Work out the finished part from the listing and answer in its coordinate system (mm). Give positions to 0.01 mm unless a question says otherwise; leave off trailing zeros. Loops run counter-clockwise (first coordinate to the right, second up) from the corner with the lowest first, then second, coordinate; pieces in that order, holes last. Notation, with made-up numbers: M 15.25,81.5 L 70.25,81.5 A8 cw 70.25,93.5 Z; hole C 55,15.25 d7. An arc over 180 degrees is marked long. Write item = value, one per line. Start each with the question number.
1. Section A-A on z = 4.5 is taken. Determine the outline of the cut face in (x, y), plus the area to 3 significant figures.
2. The mould has two halves that part along X. Classify faces 1 (the face through (70, 1, 2)), 2 (the face through (1, 0, -4)), 3 (the face through (-60.97, 1.52, 24.79)), 4 (the face through (-70, 1, 2)): released by +X, released by -X, zero draft, split by the parting line, or undercut.
3. Section C-C on y = 1 is taken. Determine the outline of the cut face in (x, z), plus the area to 3 significant figures.
4. A flat-ended cylindrical pin translates along its axis: pin 1 Ø3.5 at (x, z) = (63, 27) entering from -Y. Find the tip coordinate at first contact, or state that the pin passes through.
5. Section D-D on x = -63 is taken. Determine the outline of the cut face in (y, z).
6. Section B-B on x = 20 is taken. Determine the outline of the cut face in (y, z), plus the area to 3 significant figures.
7. Consider L1, parallel to X at y = 0.7, z = 4.5; L2, parallel to X at y = 1.5, z = -25; L3, parallel to Z at x = -35, y = 0.9. Determine where each line is inside the solid, lowest interval first. Write a range as [from, to].
```python
from build123d import *

# Parameters (mm, degrees)
BOSS_EXTRUDE1_DEPTH = 3
SKETCH3_R           = 3
CUT_EXTRUDE1_DEPTH  = 10
SKETCH4_R           = 4.62
CUT_EXTRUDE2_DEPTH  = 10


with BuildPart() as part:
    # Sketch1 → Boss-Extrude1 (new body)
    with BuildSketch(Plane(origin=(0, 0, 0), x_dir=(1, 0, 0), z_dir=(0, 1, 0))):
        with BuildLine():
            Line((70, 28.5), (70, -32.5))
            Line((70, -32.5), (-70, -32.5))
            Line((-70, -32.5), (-70, 28.5))
            ThreePointArc((-70, 28.5), (0, 38.554020598), (70, 28.5))
        make_face()
    extrude(amount=BOSS_EXTRUDE1_DEPTH)

    # Sketch3 → Cut-Extrude1 (cut)
    with BuildSketch(Plane(origin=(0, 3, 0), x_dir=(1, 0, 0), z_dir=(0, 1, 0))):
        with Locations(Location((-63, 25, 0), (0, 0, 270))):
            Circle(SKETCH3_R)
        with Locations(Location((-63, -27, 0), (0, 0, 270))):
            Circle(SKETCH3_R)
        with Locations(Location((63, 25, 0), (0, 0, 270))):
            Circle(SKETCH3_R)
        with Locations(Location((63, -27, 0), (0, 0, 270))):
            Circle(SKETCH3_R)
    extrude(amount=-CUT_EXTRUDE1_DEPTH, mode=Mode.SUBTRACT)

    # Sketch4 → Cut-Extrude2 (cut)
    with BuildSketch(Plane(origin=(0, 0, 0), x_dir=(-1, 0, 0), z_dir=(0, -1, 0))):
        with Locations(Location((23.33, -4.5, 0), (0, 0, 90))):
            Circle(SKETCH4_R)
        with Locations(Location((-22.67, -4.5, 0), (0, 0, 90))):
            Circle(SKETCH4_R)
        with Locations(Location((-0.055991236, 20.138512818, 0), (0, 0, 90))):
            Circle(SKETCH4_R)
    extrude(amount=-CUT_EXTRUDE2_DEPTH, mode=Mode.SUBTRACT)


solid = part.part
```
Verdict:
q1.outline = M -70,0 L -27.95,0 L -27.95,3 L -70,3 Z; M -18.71,0 L 18.05,0 L 18.05,3 L -18.71,3 Z; M 27.29,0 L 70,0 L 70,3 L 27.29,3 Z
q1.area = 365 mm2
q2.face_1 = released by +X
q2.face_2 = zero draft
q2.face_3 = undercut
q2.face_4 = released by -X
q3.outline = M -70,-28.5 A248.71 ccw 70,-28.5 L 70,32.5 L -70,32.5 Z; hole C -63,-25 d6; hole C -63,27 d6; hole C -23.33,4.5 d9.24; hole C 0.06,-20.14 d9.24; hole C 22.67,4.5 d9.24; hole C 63,-25 d6; hole C 63,27 d6
q3.area = 9,170 mm2
q4.pin_1 = through
q5.outline = M 0,-30.44 L 3,-30.44 L 3,-28 L 0,-28 Z; M 0,-22 L 3,-22 L 3,24 L 0,24 Z; M 0,30 L 3,30 L 3,32.5 L 0,32.5 Z
q6.outline = M 0,-37.75 L 3,-37.75 L 3,0.73 L 0,0.73 Z; M 0,8.27 L 3,8.27 L 3,32.5 L 0,32.5 Z
q6.area = 188 mm2
q7.L1 = [-70, -27.95], [-18.71, 18.05], [27.29, 70]
q7.L2 = [-70, -66], [-60, 60], [66, 70]
q7.L3 = [-36.08, 32.5]
